Geometry: see drawing. Coordinates: mm, zero at the bounding-box minimum. A direction names the side the tool comes from. Round coordinates to 2 decimals unless told otherwise and drop trailing zeros. Write each loop counter-clockwise with the first axis right and the second up, starting at its lowest first coordinate (ties: lowest second). Pieces come first, ordered by that corner, then holes. Notation, with made-up numbers: M 74,30.25 L 106,30.25 A33 ccw 106,63.25 Z; hole C 28.5,-13.75 d2. An arc over 180 degrees is marked long. Use a Markdown table: item, result.
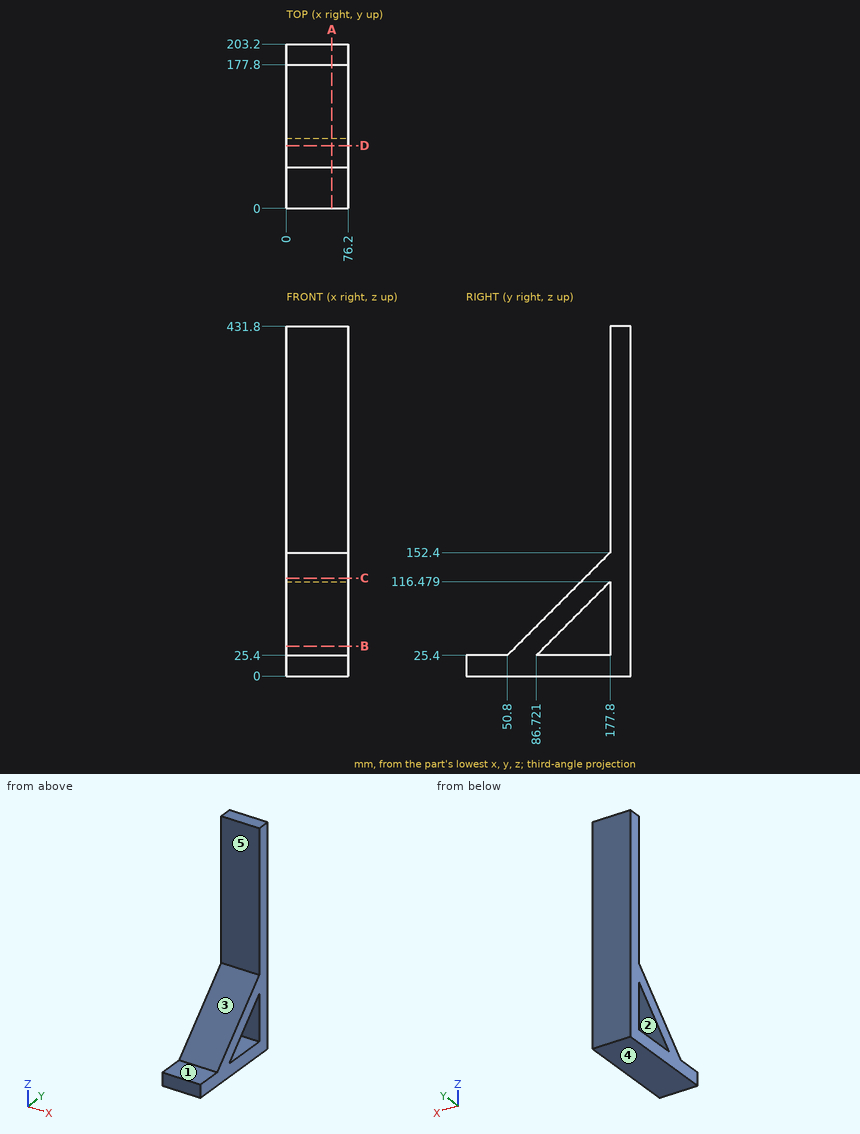
Q1. Reachability of the marked faces 4 and 5 from +Z, -Z, +X, -X, +Y, -Y: full face, straight path, thin tool, end or side. Return the list, or none.
Results are:
| item | result |
|---|---|
| face 4 | -Z, +X, -X, +Y, -Y |
| face 5 | +Z, +X, -X, -Y |
Q2. Mould query, pull axis Y, two halves, no side actions, for the marked faces 1, 2 and 3. Classes: +Y half, -Y half, draft (parallel to the pull), parting line (faces both ways), or undercut.
Results are:
| item | result |
|---|---|
| face 1 | draft |
| face 2 | undercut |
| face 3 | -Y half |
Q3. Line query: L1, parallel to Z at x = 25, y = 34; L2, parallel to Y at x = 57, z = 349; L3, parallel to Y at x = 59, z = 78.5. Output: solid intervals per line, ascending.
Results are:
| item | result |
|---|---|
| L1 | 0 to 25.4 |
| L2 | 177.8 to 203.2 |
| L3 | 103.9 to 139.82, 177.8 to 203.2 |
Q4. Section A-A on x = 56. Return loops of the section in (y, z).
Results are:
| item | result |
|---|---|
| outline | M 0,0 L 203.2,0 L 203.2,431.8 L 177.8,431.8 L 177.8,152.4 L 50.8,25.4 L 0,25.4 Z; hole M 86.72,25.4 L 177.8,25.4 L 177.8,116.48 Z |
Q5. Section C-C on z = 121. Return loops of the section in (x, y).
Results are:
| item | result |
|---|---|
| outline | M 0,146.4 L 76.2,146.4 L 76.2,203.2 L 0,203.2 Z |
Q6. Section D-D on y = 77.5. Return loops of the section in (x, z).
Results are:
| item | result |
|---|---|
| outline | M 0,0 L 76.2,0 L 76.2,52.1 L 0,52.1 Z |
Q7. First-contact query: pin 1 Ø23 at (x, z) = (54.5, 62.5) entering from -Y; pin 2 Ø23 at (x, y) = (42, 144.5) entering from +Z. Flat tips, straight axial feed; report the tip coordinate or a pass-through.
Results are:
| item | result |
|---|---|
| pin 1 | y = 76.4 |
| pin 2 | z = 130.6 |
Q8. Section B-B on z = 37. Return loops of the section in (x, y).
Results are:
| item | result |
|---|---|
| outline | M 0,62.4 L 76.2,62.4 L 76.2,98.32 L 0,98.32 Z; M 0,177.8 L 76.2,177.8 L 76.2,203.2 L 0,203.2 Z |
